Design review of the part built by this model. Coordinates are the model's own, in mm. Face numbers are marked on the shaded views. Give positions to 0.01 mm unless a question says otherwise; leave off trailing zeros. Loops run counter-clockwise (first coordinate to the right, second up) from the corner with the lowest first, then second, coordinate; pieces in that order, holes last. Notation, with made-up numbers: (-36, 51) -> (-9, 51) arc R33 ccw to (-9, 86) -> close; hole circle Ø6 at (69.25, -12.5). An arc over 180 degrees is marked (long way). Answer as CSV lines item,"result".
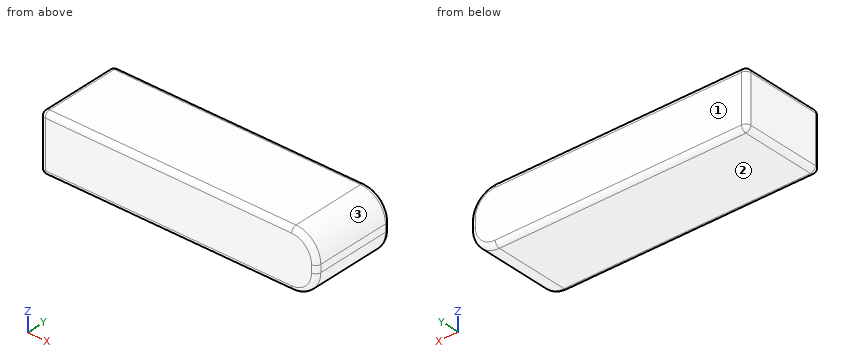
Autodesk Inventor part; units mm, degrees
ref_plane "YZ Plane" through (0, 0, 0) normal (1, 0, 0) x (0, 1, 0)
ref_plane "XZ Plane" through (0, 0, 0) normal (0, 1, 0) x (-1, 0, 0)
ref_plane "XY Plane" through (0, 0, 0) normal (0, 0, 1) x (1, 0, 0)
sketch "スケッチ1" plane through (0, 0, 0) normal (0, 0, 1) x (1, 0, 0)
  line L0 (-55.5, 17) -> (55.5, 17)
  line L1 (55.5, 17) -> (55.5, -17)
  line L2 (55.5, -17) -> (-55.5, -17)
  line L3 (-55.5, -17) -> (-55.5, 17)
  line L4 (-55.5, 17) -> (55.5, -17) construction
  line L5 (55.5, 17) -> (-55.5, -17) construction
  point P0 (0, 0)
  dimension "d0" = 111
  dimension "d1" = 34
extrude "押し出し1" add sketch "スケッチ1" along normal blind 23
fillet "フィレット1" radius 10 2 edges at (55.5, 0, 23) (55.5, 0, 0)
fillet "フィレット2" radius 2 14 edges at (-55.5, 0, 23) (-55.5, 17, 11.5) (-55.5, 0, 0) (-55.5, -17, 11.5) (52.5711, 17, 20.0711) (55.5, 17, 11.5) (52.5711, 17, 2.9289) (-5, 17, 0) (-5, 17, 23) (52.5711, -17, 20.0711) (55.5, -17, 11.5) (52.5711, -17, 2.9289) (-5, -17, 0) (-5, -17, 23)
properties part number "HP-G830C2800S3"
Q1. We need section A-A, the plane y = 4. State the section outline as (x, z) points, and give its area (3 significant figures).
Filled sheet:
outline,"(-55.5, 2) arc R2 ccw to (-53.5, 0) -> (45.5, 0) arc R10 ccw to (55.5, 10) -> (55.5, 13) arc R10 ccw to (45.5, 23) -> (-53.5, 23) arc R2 ccw to (-55.5, 21) -> close"
area,"2,510 mm^2"
Q2. The part is to be moulded in two halves that separate along Z. For the marked faces 1, 2 and 3, say which applies: pulls with the +Z half, pulls with the -Z half, needs draft (parallel to the pull), parting line crosses it, or undercut.
Filled sheet:
face 1,"needs draft"
face 2,"pulls with the -Z half"
face 3,"pulls with the +Z half"
Q3. Clearance check with a flat-ended pin moving along its axis: pin 1 Ø1 at (y, z) = (-8, 17) entering from +X. State where the tip first meets the part, or that it passes through.
Filled sheet:
pin 1,"stops at x = 54.87"
Q4. To check wall thickness, follow probe 1 along Y at (x, z) = (5, 21.25); probe 2 along X at (y, z) = (-8, 9.75); probe 3 along X at (y, z) = (8.5, 20.75). State the ranges of each line that lie inside material, in increasing order. Write a range as from..to.
Filled sheet:
probe 1,"y = -16.98..16.98"
probe 2,"x = -55.5..55.5"
probe 3,"x = -55.5..51.82"
